```python
from build123d import *

# Parameters (mm, degrees)
F1_DEPTH = 38.1
F2_R     = 6.35
F3_R     = 15.875
F4_R     = 7.9375
F5_DEPTH = 25.4
F6_W     = 711.2
F6_H     = 101.6
F6_R     = 7.9375
F7_DEPTH = 3.175


with BuildPart() as f1:
    # F0 (on Front) → F1 (new body, symmetric)
    with BuildSketch(Plane.XZ):
        with BuildLine():
            Line((255.5875, -254), (341.3125, -254))
            Line((341.3125, -254), (341.3125, -244.475))
            Line((341.3125, -244.475), (265.1125, -244.475))
            Line((265.1125, -244.475), (265.1125, 0))
            ThreePointArc((265.1125, 0), (0, 265.1125), (-265.1125, 0))
            Line((-265.1125, 0), (-265.1125, -244.475))
            Line((-265.1125, -244.475), (-341.3125, -244.475))
            Line((-341.3125, -244.475), (-341.3125, -254))
            Line((-341.3125, -254), (-255.5875, -254))
            Line((-255.5875, -254), (-255.5875, 0))
            ThreePointArc((-255.5875, 0), (0, 255.5875), (255.5875, 0))
            Line((255.5875, 0), (255.5875, -254))
        make_face()
    extrude(amount=F1_DEPTH, both=True)

    # F2
    f2_edges = [f1.edges().sort_by_distance(p)[0] for p in [
        (-265.1125, 0, -244.475),
        (265.1125, 0, -244.475),
    ]]
    fillet(f2_edges, radius=F2_R)

    # F3
    f3_edges = [f1.edges().sort_by_distance(p)[0] for p in [
        (-255.5875, 0, -254),
        (255.5875, 0, -254),
    ]]
    fillet(f3_edges, radius=F3_R)

    # F4 (on face) → F5 (cut)
    with BuildSketch(Plane(origin=(0, 0, -254), x_dir=(1, 0, 0), z_dir=(0, 0, -1))):
        with Locations((-304.8, 0)):
            Circle(F4_R)
        with Locations((304.8, 0)):
            Circle(F4_R)
    extrude(amount=-F5_DEPTH, mode=Mode.SUBTRACT)

    # F6 (on face) → F7 (join)
    with BuildSketch(Plane(origin=(0, 0, -254), x_dir=(1, 0, 0), z_dir=(0, 0, -1))):
        Rectangle(F6_W, F6_H)
        with Locations((-304.8, 0)):
            Circle(F6_R, mode=Mode.SUBTRACT)
        with Locations((304.8, 0)):
            Circle(F6_R, mode=Mode.SUBTRACT)
    extrude(amount=F7_DEPTH)


solid = f1.part
```
Geometry check sheet. Reference: the model listing, model coordinates, mm. A direction names the side the tool comes from. Coordinates: 2 decimals unless noted, no trailing zeros. Loops run counter-clockwise (first coordinate to the right, second up) from the corner with the lowest first, then second, coordinate; pieces in that order, holes last. Notation, with made-up numbers: (80, 65) -> (95, 65) arc R30 ccw to (95, 99) -> close; hole circle Ø11 at (18.25, 63). An arc over 180 degrees is marked (long way). Put each result on its own line as item: value.
1) Cross-section at D-D on x = 304.8. Record the boundary of the cut face in (y, z) (1 decimal), plus the area to 3 significant figures.
Result set:
outline: (-50.8, -257.2) -> (-7.9, -257.2) -> (-7.9, -244.5) -> (-38.1, -244.5) -> (-38.1, -254) -> (-50.8, -254) -> close; (7.9, -257.2) -> (50.8, -257.2) -> (50.8, -254) -> (38.1, -254) -> (38.1, -244.5) -> (7.9, -244.5) -> close
area: 847 mm^2
2) Cross-section at B-B on y = 0. Count the separate pieces of the cut face and the enclosed holes in it, plus the area to 3 significant figures.
Result set:
separate pieces: 3
enclosed holes: 1
area: 15,800 mm^2
3) Cross-section at C-C on x = 0. Record the boundary of the cut face in (y, z) (1 decimal), plus the area to 3 significant figures.
Result set:
outline: (-50.8, -257.2) -> (50.8, -257.2) -> (50.8, -254) -> (-50.8, -254) -> close; (-38.1, 255.6) -> (38.1, 255.6) -> (38.1, 265.1) -> (-38.1, 265.1) -> close
area: 1,050 mm^2
4) Thickness scan on line 1 (X direction, y = 0, z = -256); line 2 (X direction, y = 0, z = -251); line 3 (X direction, y = 0, z = -251.75). Record the ranges inside material, lowest first.
Result set:
line 1: x = -355.6 to -312.74, -296.86 to 296.86, 312.74 to 355.6
line 2: x = -341.31 to -312.74, -296.86 to -262.18, 262.18 to 296.86, 312.74 to 341.31
line 3: x = -341.31 to -312.74, -296.86 to -263.32, 263.32 to 296.86, 312.74 to 341.31
5) Release check for a two-part mould opening along X. For faces 4 (the cylindrical face through (260.36, 0.53, -249.47)), 5 (the flat face through (-2, -38.1, 257)), 6 (the cylindrical face through (5.83, -0.53, 265.05)) record: released by +X, released by -X, zero draft, split by the parting line, or undercut.
Result set:
face 4: undercut
face 5: zero draft
face 6: split by the parting line
6) Cross-section at A-A on z = -171. Record the boundary of the cut face in (x, y), plus the area to 3 significant figures.
Result set:
outline: (-265.11, -38.1) -> (-255.59, -38.1) -> (-255.59, 38.1) -> (-265.11, 38.1) -> close; (255.59, -38.1) -> (265.11, -38.1) -> (265.11, 38.1) -> (255.59, 38.1) -> close
area: 1,450 mm^2
7) Tool access check on faces 1 (the flat face through (315, -1, -244.475)), 2 (the flat face through (255.588, -1, -117)), 3 (the flat face through (-2, 38.1, 257)). Record the directions out of +Z, -Z, +X, -X, +Y, -Y that give a thin tool (end or side, any length) a straight path to the whole face; none if there is none.
Result set:
face 1: +Z, +X, +Y, -Y
face 2: +Y, -Y
face 3: +Z, +X, -X, +Y
8) Gauge pin test, flat ends, axial feed: pin 1 Ø3 at (y, z) = (-2, -247) entering from -X; pin 2 Ø1.5 at (y, z) = (-32.5, -71.5) entering from -X; pin 3 Ø12.5 at (x, y) = (-304.8, 0) entering from +Z; pin 4 Ø8 at (y, z) = (-14, 103) entering from -X. Record the tip position at first contact, or that the pin passes through.
Result set:
pin 1: stops at x = -341.31
pin 2: stops at x = -265.11
pin 3: passes through
pin 4: stops at x = -245.93
